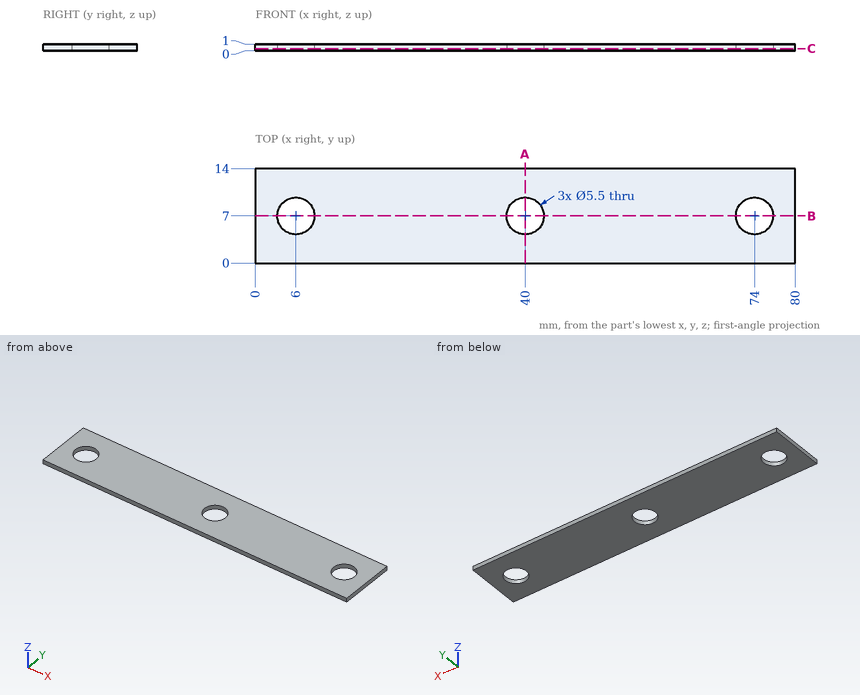
Design review of the part shown in the three views and the two pictorial views. Dimensions are in mm from the part's minimum x, y and z. Give positions to 0.01 mm unless a question says otherwise; leave off trailing zeros. Write each loop counter-clockwise with the first axis right and the second up, starting at its lowest first coordinate (ties: lowest second). Pieces come first, ordered by that corner, then holes. Notation, with made-up numbers: M -24.75,42 L -14.75,42 A25 cw -14.75,60 Z; hole C -19,78.25 d6. An arc over 180 degrees is marked long. Return JSON: item names as keys, results as strings. Group by question number.
Item 1: Wall thickness on line 1 along X through (y, z) = (7, 0.3); line 2 along X through (y, z) = (5, 0.2); line 3 along Y through (x, z) = (74, 0.5): over which ranges is each line inside the solid? List them lowest first.
Item 2: Take a section at B-B (y = 7). Give the boundary of the cut face in (x, z).
Item 3: Take a section at A-A (x = 40). Give the boundary of the cut face in (y, z), plus the area to 3 significant figures.
Item 4: Take a section at C-C (z = 0.3). Give the boundary of the cut face in (x, y), plus the area to 3 significant figures.
Return value:
{
 "1": {"line 1": "x = 0 to 3.25, 8.75 to 37.25, 42.75 to 71.25, 76.75 to 80", "line 2": "x = 0 to 4.11, 7.89 to 38.11, 41.89 to 72.11, 75.89 to 80", "line 3": "y = 0 to 4.25, 9.75 to 14"},
 "2": {"outline": "M 0,0 L 3.25,0 L 3.25,1 L 0,1 Z; M 8.75,0 L 37.25,0 L 37.25,1 L 8.75,1 Z; M 42.75,0 L 71.25,0 L 71.25,1 L 42.75,1 Z; M 76.75,0 L 80,0 L 80,1 L 76.75,1 Z"},
 "3": {"outline": "M 0,0 L 4.25,0 L 4.25,1 L 0,1 Z; M 9.75,0 L 14,0 L 14,1 L 9.75,1 Z", "area": "8.50 mm2"},
 "4": {"outline": "M 0,0 L 80,0 L 80,14 L 0,14 Z; hole C 6,7 d5.5; hole C 40,7 d5.5; hole C 74,7 d5.5", "area": "1,050 mm2"}
}
